Model file for the job. Use its own axes, mm. Face numbers are marked on the shaded views. A direction names the side the tool comes from. Coordinates: 2 decimals unless noted, no trailing zeros. Loops run counter-clockwise (first coordinate to the right, second up) from the corner with the lowest first, then second, coordinate; pieces in that order, holes last. Notation, with made-up numbers: (59, 46) -> (95, 46) arc R26 ccw to (95, 69) -> close; hole circle Ø3 at (59, 56.5). An arc over 180 degrees is marked (long way). Use one line per item in the form item = value.
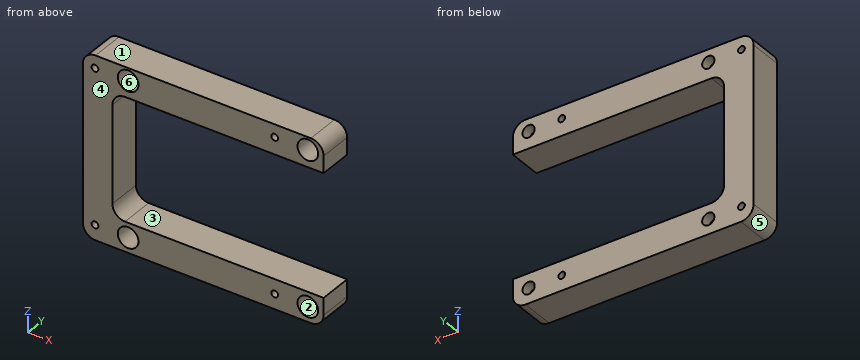
```python
from build123d import *

# Parameters (mm, degrees)
SKETCH1_W                      = 57
SKETCH1_H                      = 43
BOSS_EXTRUDE1_DEPTH            = 8
SKETCH2_W                      = 50
SKETCH2_H                      = 29
CUT_EXTRUDE1_DEPTH             = 8
FILLET1_R                      = 3
M2X0_4_TAPPED_HOLE1_D          = 1.6
CBORE_FOR_M2_SHCS1_D           = 2.9
CBORE_FOR_M2_SHCS1_CBORE_D     = 4.9
CBORE_FOR_M2_SHCS1_CBORE_DEPTH = 5.5


with BuildPart() as part:
    # Sketch1 → Boss-Extrude1 (new body)
    with BuildSketch(Plane(origin=(0, 0, 0), x_dir=(1, 0, 0), z_dir=(0, 1, 0))):
        Rectangle(SKETCH1_W, SKETCH1_H)
    extrude(amount=BOSS_EXTRUDE1_DEPTH)

    # Sketch2 → Cut-Extrude1 (cut)
    with BuildSketch(Plane(origin=(0, 0, 0), x_dir=(1, 0, 0), z_dir=(0, 1, 0))):
        with Locations((3.5, 0)):
            Rectangle(SKETCH2_W, SKETCH2_H)
    extrude(amount=CUT_EXTRUDE1_DEPTH, mode=Mode.SUBTRACT)

    # Fillet1
    fillet1_edges = [part.edges().sort_by_distance(p)[0] for p in [
        (-21.5, 4, -14.5),
        (-21.5, 4, 14.5),
        (-28.5, 4, -21.5),
        (-28.5, 4, 21.5),
        (28.5, 4, 21.5),
        (28.5, 4, -21.5),
    ]]
    fillet(fillet1_edges, radius=FILLET1_R)

    # M2x0.4 Tapped Hole1 (through all)
    with Locations(Plane(origin=(0, 0, 0), x_dir=(-1, 0, 0), z_dir=(0, -1, 0))):
        with Locations((25.63, 17.95), (25.63, -18.5), (-16.92, -18.5), (-16.92, 17.95)):
            Hole(M2X0_4_TAPPED_HOLE1_D / 2)

    # CBORE for M2 SHCS1 (through all)
    with Locations(Plane(origin=(0, 0, 0), x_dir=(-1, 0, 0), z_dir=(0, -1, 0))):
        with Locations((-24.77, 17.95), (17.78, 17.95), (17.78, -18.5), (-24.77, -18.5)):
            CounterBoreHole(CBORE_FOR_M2_SHCS1_D / 2, CBORE_FOR_M2_SHCS1_CBORE_D / 2, CBORE_FOR_M2_SHCS1_CBORE_DEPTH)


solid = part.part
```
Q1. Band-saw the part on B-B, the plane y = 6.5. State how many separate pieces and enclosed holes the cut face has, and give its area (3 significant figures).
Result:
separate_pieces = 1
enclosed_holes = 8
area = 963 mm2
Q2. Wall check: line 1 along X through (y, z) = (6.7, -17.95); line 2 along X through (y, z) = (1.65, 18.5); line 3 along Z through (x, y) = (24.77, 3.3). Give the ranges that are in metal, low to high.
Result:
line_1 = -28.5 to -26.43, -24.83 to -19.23, -16.33 to 16.12, 17.72 to 23.32, 26.22 to 28.5
line_2 = -28.5 to -26.43, -24.83 to -20.23, -15.33 to 16.12, 17.72 to 22.32, 27.22 to 28.5
line_3 = -21.5 to -20.4, -15.5 to -14.5, 14.5 to 16.05, 20.95 to 21.5
Q3. Which spindle directions (+Z, -Z, +X, -X, +Y, -Y) get a long thin tool onto all of the face, cutting with end or side? Do the marked faces 1, 2 and 3. Say none if no direction does.
Result:
face_1 = +Z, +X, -X, +Y, -Y
face_2 = -Y
face_3 = +X, +Y, -Y
Q4. Pin check, flat tips, straight feed: pin 1 Ø1.3 at (x, z) = (-25.63, 18.5) entering from -Y; pin 2 Ø2.5 at (x, z) = (-17, 17.5) entering from -Y; pin 3 Ø1 at (y, z) = (5, -6) entering from +X; pin 4 Ø1.5 at (x, z) = (26, 19) entering from -Y. Stop position of each tip, or through.
Result:
pin_1 = through
pin_2 = 0
pin_3 = -21.5
pin_4 = 5.5
Q5. Mould opens along Z. For the marked faces 4, 5 and 6 say: released by +Z, released by -Z, zero draft, split by the parting line, or undercut.
Result:
face_4 = zero draft
face_5 = released by -Z
face_6 = undercut
Q6. Band-saw the part on C-C, the plane x = -10. Write the cut outline in (y, z), and give its area (3 significant figures).
Result:
outline = (0, -21.5) -> (8, -21.5) -> (8, -14.5) -> (0, -14.5) -> close; (0, 14.5) -> (8, 14.5) -> (8, 21.5) -> (0, 21.5) -> close
area = 112 mm2
Q7. Band-saw the part on A-A, the plane x = 16.92. Write the cut outline in (y, z).
Result:
outline = (0, -21.5) -> (8, -21.5) -> (8, -18.75) -> (0, -18.75) -> close; (0, -17.15) -> (8, -17.15) -> (8, -14.5) -> (0, -14.5) -> close; (0, 14.5) -> (8, 14.5) -> (8, 17.7) -> (0, 17.7) -> close; (0, 19.3) -> (8, 19.3) -> (8, 21.5) -> (0, 21.5) -> close
Q8. Band-saw the part on D-D, the plane x = -17.78. Write the cut outline in (y, z).
Result:
outline = (0, -21.5) -> (8, -21.5) -> (8, -19.4) -> (5.5, -19.4) -> (5.5, -20.4) -> (0, -20.4) -> close; (0, -15.5) -> (5.5, -15.5) -> (5.5, -16.5) -> (8, -16.5) -> (8, -14.5) -> (0, -14.5) -> close; (0, 14.5) -> (8, 14.5) -> (8, 17.05) -> (5.5, 17.05) -> (5.5, 16.05) -> (0, 16.05) -> close; (0, 20.95) -> (5.5, 20.95) -> (5.5, 19.95) -> (8, 19.95) -> (8, 21.5) -> (0, 21.5) -> close
